from build123d import *
from OCP.BRepFilletAPI import BRepFilletAPI_MakeChamfer

# Parameters (mm, degrees)
SKETCH1_W           = 68.58
SKETCH1_H           = 38.608
BOSS_EXTRUDE1_DEPTH = 1.27
SKETCH2_W           = 68.58
SKETCH2_H           = 1.27
BOSS_EXTRUDE2_DEPTH = 9.144
SKETCH4_W           = 1.27
SKETCH4_H           = 36.068
BOSS_EXTRUDE4_DEPTH = 2.54
CHAMFER2_SIZE       = 6.604
CHAMFER2_SIZE_2     = 2.540000001


with BuildPart() as part:
    # Sketch1 → Boss-Extrude1 (new body)
    with BuildSketch(Plane(origin=(0, 0, 0), x_dir=(1, 0, 0), z_dir=(0, 1, 0))):
        with Locations((34.29, 19.304)):
            Rectangle(SKETCH1_W, SKETCH1_H)
    extrude(amount=BOSS_EXTRUDE1_DEPTH)

    # Sketch2 → Boss-Extrude2 (add)
    with BuildSketch(Plane(origin=(0, 1.27, 0), x_dir=(1, 0, 0), z_dir=(0, 1, 0))):
        with Locations((34.29, 37.973)):
            Rectangle(SKETCH2_W, SKETCH2_H)
        with Locations((34.29, 0.635)):
            Rectangle(SKETCH2_W, SKETCH2_H)
    extrude(amount=BOSS_EXTRUDE2_DEPTH)

    # Sketch4 → Boss-Extrude4 (add)
    with BuildSketch(Plane(origin=(0, 1.27, 0), x_dir=(1, 0, 0), z_dir=(0, 1, 0))):
        with Locations((0.635, 19.304)):
            Rectangle(SKETCH4_W, SKETCH4_H)
        with Locations((23.071666667, 19.304)):
            Rectangle(SKETCH4_W, SKETCH4_H)
        with Locations((45.508333333, 19.304)):
            Rectangle(SKETCH4_W, SKETCH4_H)
        with Locations((67.945, 19.304)):
            Rectangle(SKETCH4_W, SKETCH4_H)
    extrude(amount=BOSS_EXTRUDE4_DEPTH)

    # Chamfer2
    chamfer2_edges_1 = [part.edges().sort_by_distance(p)[0] for p in [
        (67.945, 3.81, -37.338),
    ]]
    chamfer2_side_1 = [part.faces().sort_by_distance(p)[0] for p in [
        (67.945, 3.8608, -37.338),
    ]]
    chamfer2_edges_2 = [part.edges().sort_by_distance(p)[0] for p in [
        (45.508333333, 3.81, -37.338),
    ]]
    chamfer2_side_2 = [part.faces().sort_by_distance(p)[0] for p in [
        (45.508333333, 3.8608, -37.338),
    ]]
    chamfer2_edges_3 = [part.edges().sort_by_distance(p)[0] for p in [
        (23.071666667, 3.81, -37.338),
    ]]
    chamfer2_side_3 = [part.faces().sort_by_distance(p)[0] for p in [
        (23.071666667, 3.8608, -37.338),
    ]]
    chamfer2_edges_4 = [part.edges().sort_by_distance(p)[0] for p in [
        (0.635, 3.81, -37.338),
    ]]
    chamfer2_side_4 = [part.faces().sort_by_distance(p)[0] for p in [
        (0.635, 3.8608, -37.338),
    ]]
    chamfer2_edges_5 = [part.edges().sort_by_distance(p)[0] for p in [
        (67.945, 3.81, -1.27),
    ]]
    chamfer2_side_5 = [part.faces().sort_by_distance(p)[0] for p in [
        (67.945, 3.8608, -1.27),
    ]]
    chamfer2_edges_6 = [part.edges().sort_by_distance(p)[0] for p in [
        (45.508333333, 3.81, -1.27),
    ]]
    chamfer2_side_6 = [part.faces().sort_by_distance(p)[0] for p in [
        (45.508333333, 3.8608, -1.27),
    ]]
    chamfer2_edges_7 = [part.edges().sort_by_distance(p)[0] for p in [
        (23.071666667, 3.81, -1.27),
    ]]
    chamfer2_side_7 = [part.faces().sort_by_distance(p)[0] for p in [
        (23.071666667, 3.8608, -1.27),
    ]]
    chamfer2_edges_8 = [part.edges().sort_by_distance(p)[0] for p in [
        (0.635, 3.81, -1.27),
    ]]
    chamfer2_side_8 = [part.faces().sort_by_distance(p)[0] for p in [
        (0.635, 3.8608, -1.27),
    ]]
    chamfer2 = BRepFilletAPI_MakeChamfer(part.part.solid().wrapped)
    for e in chamfer2_edges_1:
        chamfer2.Add(CHAMFER2_SIZE - 0.0001, CHAMFER2_SIZE_2 - 0.0001, e.wrapped, chamfer2_side_1[0].wrapped)
    for e in chamfer2_edges_2:
        chamfer2.Add(CHAMFER2_SIZE - 0.0001, CHAMFER2_SIZE_2 - 0.0001, e.wrapped, chamfer2_side_2[0].wrapped)
    for e in chamfer2_edges_3:
        chamfer2.Add(CHAMFER2_SIZE - 0.0001, CHAMFER2_SIZE_2 - 0.0001, e.wrapped, chamfer2_side_3[0].wrapped)
    for e in chamfer2_edges_4:
        chamfer2.Add(CHAMFER2_SIZE - 0.0001, CHAMFER2_SIZE_2 - 0.0001, e.wrapped, chamfer2_side_4[0].wrapped)
    for e in chamfer2_edges_5:
        chamfer2.Add(CHAMFER2_SIZE - 0.0001, CHAMFER2_SIZE_2 - 0.0001, e.wrapped, chamfer2_side_5[0].wrapped)
    for e in chamfer2_edges_6:
        chamfer2.Add(CHAMFER2_SIZE - 0.0001, CHAMFER2_SIZE_2 - 0.0001, e.wrapped, chamfer2_side_6[0].wrapped)
    for e in chamfer2_edges_7:
        chamfer2.Add(CHAMFER2_SIZE - 0.0001, CHAMFER2_SIZE_2 - 0.0001, e.wrapped, chamfer2_side_7[0].wrapped)
    for e in chamfer2_edges_8:
        chamfer2.Add(CHAMFER2_SIZE - 0.0001, CHAMFER2_SIZE_2 - 0.0001, e.wrapped, chamfer2_side_8[0].wrapped)
    add(Compound.cast(chamfer2.Shape()), mode=Mode.REPLACE)  # a hair under: the kernel refuses the full size


solid = part.part
Design review of the part built by this model. Coordinates are the model's own, in mm. A direction names the side the tool comes from. Round coordinates to 2 decimals unless told otherwise and drop trailing zeros. Write each loop counter-clockwise with the first axis right and the second up, starting at its lowest first coordinate (ties: lowest second). Pieces come first, ordered by that corner, then holes. Notation, with made-up numbers: (56.25, 78.5) - (71.25, 78.5) arc R7 ccw to (71.25, 86.5) - close; hole circle Ø6 at (-14.75, -3). An arc over 180 degrees is marked (long way). Use a Markdown table: item, result. Add a question column.
1. For faces 1 (the face through (68, 3.81, -20)), 2 (the face through (34, 5, 0)), 3 (the face through (12, 1.27, -20)), list the 3-axis set-ups (+Z, -Z, +X, -X, +Y, -Y) from which the entire face can be reached by the end or side of a thin tool; tool diameter is ignored.
2. Wall thickness on probe 1 along X at (y, z) = (2.25, -4.5); probe 2 along Z at (x, y) = (31, 9); probe 3 along Y at (x, z) = (51, -8.5): over which ranges is each line inside the solid? List them lowest first.
3. Clearance check with flat-ended pins moving along their axes: pin 1 (6.5 mm diameter, centred on x = 36, z = -25, fed in from +Y); pin 2 (0.6 mm diameter, centred on x = 45.5, z = -12.5, fed in from +Y). State where each tip first meets the part, or that it passes through.
4. We need section C-C (x = 32). State the section outline as (y, z) points.
5. Mouldability with a two-part tool opening along X and no side actions: class faces 4 (the face through (45.5, 3.81, -19.5)), 5 (the face through (57, 1.27, -20)), 6 (the face through (0, 3, -19)) as +X half, -X half, draft (parallel to the pull), parting line (faces both ways), or undercut.
6. We need section A-A (z = -8.5). State the section outline as (x, y) points, then the cut area to 4 significant figures.
Output:
| question | item | result |
|---|---|---|
| 1 | face 1 | +X, -X, +Y |
| 1 | face 2 | +Z, +X, -X, +Y, -Y |
| 1 | face 3 | +Y |
| 2 | probe 1 | x = 0 to 1.27, 22.44 to 23.71, 44.87 to 46.14, 67.31 to 68.58 |
| 2 | probe 2 | z = -38.61 to -37.34, -1.27 to 0 |
| 2 | probe 3 | y = 0 to 1.27 |
| 3 | pin 1 | stops at y = 1.27 |
| 3 | pin 2 | stops at y = 3.81 |
| 4 | outline | (0, -38.61) - (10.41, -38.61) - (10.41, -37.34) - (1.27, -37.34) - (1.27, -1.27) - (10.41, -1.27) - (10.41, 0) - (0, 0) - close |
| 5 | face 4 | draft |
| 5 | face 5 | undercut |
| 5 | face 6 | -X half |
| 6 | outline | (0, 0) - (68.58, 0) - (68.58, 3.81) - (67.31, 3.81) - (67.31, 1.27) - (46.14, 1.27) - (46.14, 3.81) - (44.87, 3.81) - (44.87, 1.27) - (23.71, 1.27) - (23.71, 3.81) - (22.44, 3.81) - (22.44, 1.27) - (1.27, 1.27) - (1.27, 3.81) - (0, 3.81) - close |
| 6 | area | 100.0 mm2 |
